from build123d import *

# Parameters (mm, degrees)
CROQUIS2_W              = 4.2
CROQUIS2_H              = 4.2
SALIENTE_EXTRUIR1_DEPTH = 400


with BuildPart() as part:
    # Croquis2 → Saliente-Extruir1 (new body)
    with BuildSketch(Plane(origin=(0, 0, 0), x_dir=(1, 0, 0), z_dir=(0, 1, 0))):
        Polygon((-37.373217156, 24.271112291), (-26.498217156, 24.271112291), (-26.498217156, 23.171112291), (-30.573217156, 23.171112291), (-30.573217156, 19.168168566), (-26.586160881, 15.181112291), (-18.160273431, 15.181112291), (-14.173217156, 19.168168566), (-14.173217156, 23.171112291), (-18.248217156, 23.171112291), (-18.248217156, 24.271112291), (-7.373217156, 24.271112291), (-7.373217156, 13.396112291), (-8.473217156, 13.396112291), (-8.473217156, 17.471112291), (-12.476160881, 17.471112291), (-16.463217156, 13.484056016), (-16.463217156, 5.058168566), (-12.476160881, 1.071112291), (-8.473217156, 1.071112291), (-8.473217156, 5.146112291), (-7.373217156, 5.146112291), (-7.373217156, -5.728887709), (-18.248217156, -5.728887709), (-18.248217156, -4.628887709), (-14.173217156, -4.628887709), (-14.173217156, -0.625943984), (-18.160273431, 3.361112291), (-26.586160881, 3.361112291), (-30.573217156, -0.625943984), (-30.573217156, -4.628887709), (-26.498217156, -4.628887709), (-26.498217156, -5.728887709), (-37.373217156, -5.728887709), (-37.373217156, 5.146112291), (-36.273217156, 5.146112291), (-36.273217156, 1.071112291), (-32.270273431, 1.071112291), (-28.283217156, 5.058168566), (-28.283217156, 13.484056016), (-32.270273431, 17.471112291), (-36.273217156, 17.471112291), (-36.273217156, 13.396112291), (-37.373217156, 13.396112291), align=None)
        with Locations((-10.573217156, 21.071112291)):
            Rectangle(CROQUIS2_W, CROQUIS2_H, mode=Mode.SUBTRACT)
        with Locations((-34.173217156, -2.528887709)):
            Rectangle(CROQUIS2_W, CROQUIS2_H, mode=Mode.SUBTRACT)
        with Locations((-34.173217156, 21.071112291)):
            Rectangle(CROQUIS2_W, CROQUIS2_H, mode=Mode.SUBTRACT)
        with Locations((-10.573217156, -2.528887709)):
            Rectangle(CROQUIS2_W, CROQUIS2_H, mode=Mode.SUBTRACT)
        with BuildLine():
            Line((-19.165547938, 11.064567946), (-18.248217156, 11.981898728))
            Line((-18.248217156, 11.981898728), (-19.662430718, 13.396112291))
            Line((-19.662430718, 13.396112291), (-20.5797615, 12.478781509))
            ThreePointArc((-20.5797615, 12.478781509), (-22.373217156, 12.946112291), (-24.166672811, 12.478781509))
            Line((-24.166672811, 12.478781509), (-25.084003593, 13.396112291))
            Line((-25.084003593, 13.396112291), (-26.498217156, 11.981898728))
            Line((-26.498217156, 11.981898728), (-25.580886374, 11.064567946))
            ThreePointArc((-25.580886374, 11.064567946), (-26.048217156, 9.271112291), (-25.580886374, 7.477656635))
            Line((-25.580886374, 7.477656635), (-26.498217156, 6.560325853))
            Line((-26.498217156, 6.560325853), (-25.084003593, 5.146112291))
            Line((-25.084003593, 5.146112291), (-24.166672811, 6.063443073))
            ThreePointArc((-24.166672811, 6.063443073), (-22.373217156, 5.596112291), (-20.5797615, 6.063443073))
            Line((-20.5797615, 6.063443073), (-19.662430718, 5.146112291))
            Line((-19.662430718, 5.146112291), (-18.248217156, 6.560325853))
            Line((-18.248217156, 6.560325853), (-19.165547938, 7.477656635))
            ThreePointArc((-19.165547938, 7.477656635), (-18.698217156, 9.271112291), (-19.165547938, 11.064567946))
        make_face(mode=Mode.SUBTRACT)
    extrude(amount=SALIENTE_EXTRUIR1_DEPTH)


solid = part.part
Geometry: final body of the model. Coordinates: model frame, mm. Coordinates: 2 decimals unless noted, no trailing zeros.
1) Draft query along X for faces 1 (the flat face through (-22, 197, -15.181)), 2 (the flat face through (-7.373, 197, 0)), 3 (the flat face through (-22, 197, -3.361)), 4 (the flat face through (-37.373, 197, -19)). Return one class per face: released by +X, released by -X, zero draft, split by the parting line, or undercut.
Result sheet:
face 1: undercut
face 2: released by +X
face 3: undercut
face 4: released by -X
2) First-contact query: P1, Ø1.5, axis at x = -33.5, z = -16.5, coming from the +Y side (3 decimals); P2, Ø6.5, axis at x = -23, y = 181, coming from the -Z side. Flat tips, straight axial feed; report the tip coordinate or a pass-through.
Result sheet:
P1: passes through
P2: stops at z = -15.18
3) Ray query, probe 1 along X at (y, z) = (235, 3.5); probe 2 along Z at (x, y) = (-35, 180); probe 3 along X at (y, z) = (259, -5). Return the intervals inside material, ascending.
Result sheet:
probe 1: x = -37.37 to -36.27, -32.07 to -30.57, -14.17 to -12.67, -8.47 to -7.37
probe 2: z = -24.27 to -23.17, -18.97 to -17.47, -1.07 to 0.43, 4.63 to 5.73
probe 3: x = -37.37 to -36.27, -28.34 to -16.41, -8.47 to -7.37
4) Section A-A (y = 137). Give the number of separate pieces and of enclosed holes in the cut face, then the cut area to 3 significant figures.
Result sheet:
separate pieces: 1
enclosed holes: 5
area: 281 mm2
